Answer from the drawing. Dimensions are ordinates in mm from the lowest x, y and z of the part. Round coordinates to 2 decimals unless told otherwise and drop trailing zeros. Loops run counter-clockwise (first coordinate to the right, second up) from the corner with the lowest first, then second, coordinate; pieces in that order, holes last. Notation, with made-up numbers: M -30.5,-28 L 27.5,-28 A18 cw 27.5,-5 Z; hole C 15,45 d10. An arc over 180 degrees is marked long. One line per item, written item: value.
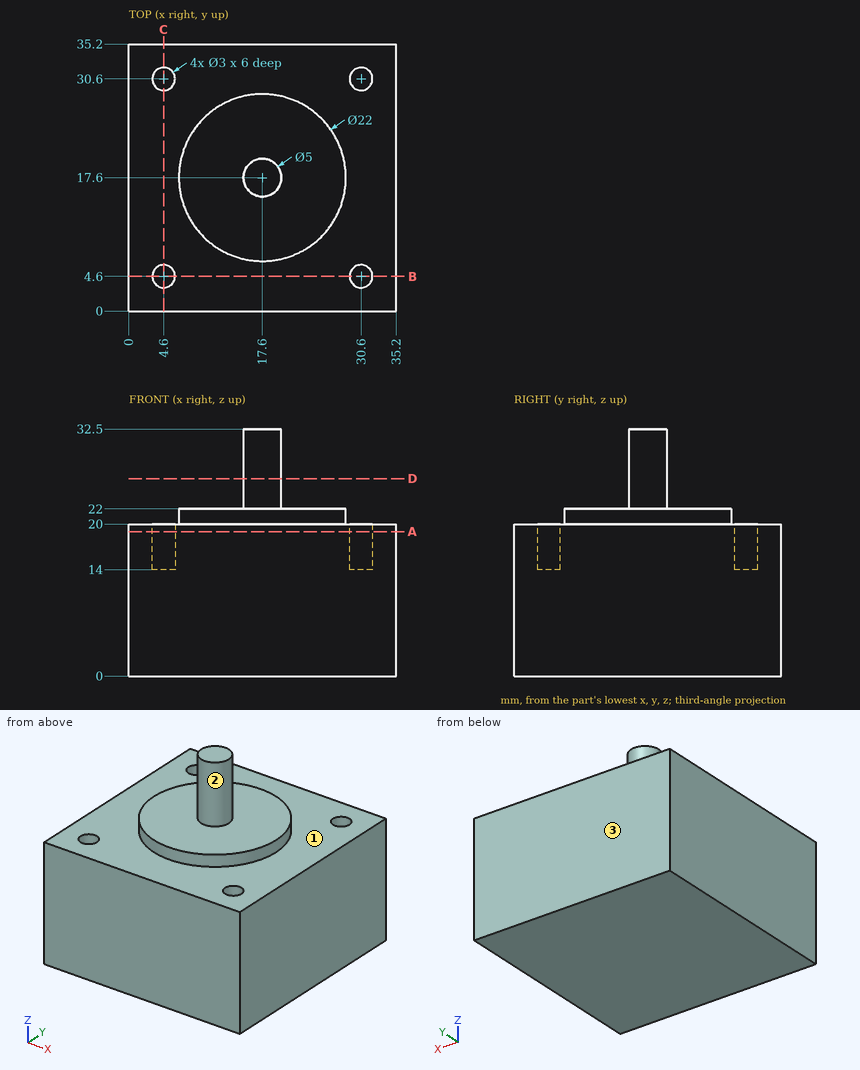
1) Find section D-D (z = 26). Give the vertices of the cut face in (x, y).
Check values:
outline: C 17.6,17.6 d5
2) Find section B-B (y = 4.6). Give the vertices of the cut face in (x, z).
Check values:
outline: M 0,0 L 35.2,0 L 35.2,20 L 32.1,20 L 32.1,14 L 29.1,14 L 29.1,20 L 6.1,20 L 6.1,14 L 3.1,14 L 3.1,20 L 0,20 Z
3) The mould has two halves that part along Y. Classify the marked faces 1, 2 and 3: +Y half, -Y half, draft (parallel to the pull), parting line (faces both ways), or undercut.
Check values:
face 1: draft
face 2: parting line
face 3: +Y half
4) Find the intervals of material crossed by probe 1 along Y at (x, z) = (30.6, 18.55); probe 2 along Y at (x, z) = (4, 15), in increasing order. Write a range as from..to.
Check values:
probe 1: 0..3.1, 6.1..29.1, 32.1..35.2
probe 2: 0..3.23, 5.97..29.23, 31.97..35.2
5) Find section A-A (z = 19). Give the vertices of the cut face in (x, y).
Check values:
outline: M 0,0 L 35.2,0 L 35.2,35.2 L 0,35.2 Z; hole C 4.6,4.6 d3; hole C 4.6,30.6 d3; hole C 30.6,4.6 d3; hole C 30.6,30.6 d3
6) Each of these flat-tipped pins is pushed along its axis until it touches: pin 1 (1.5 mm diameter, centred on x = 5.5, y = 5, fed in from +Z); pin 2 (10 mm diameter, centred on x = 23, z = 29, fed in from +Y); pin 3 (1.5 mm diameter, centred on x = 4.5, y = 30.5, fed in from +Z). Where does it stop, or does it pass through?
Check values:
pin 1: z = 20
pin 2: y = 20.07
pin 3: z = 14
